For this review, take the finished solid that the model builds, in its own axes (mm). Face numbers are marked on the shaded views. A direction names the side the tool comes from. Round coordinates to 2 decimals unless told otherwise and drop trailing zeros. Order: outer loops, then holes, each group sorted by start corner. A loop starts at its lowest first (then second) coordinate and runs counter-clockwise, first axis right, second up. Notation, with made-up numbers: (-37.75, 54) -> (6.25, 54) arc R8 ccw to (6.25, 67) -> close; hole circle Ø7 at (22, 8). An arc over 180 degrees is marked (long way). Answer in a Markdown table with one row per item.
```python
from build123d import *

# Parameters (mm, degrees)
SKETCH_1_W               = 38.5
SKETCH_1_H               = 38.5
EXTRUDE_1_DEPTH          = 6.5
SKETCH_2_W               = 2.5
SKETCH_2_H               = 4
SKETCH_2_W_2             = 6
SKETCH_2_H_2             = 6
EXTRUDE_2_DEPTH          = 2
M3X0_5_1_D               = 2.5
M3X0_5_1_DEPTH           = 7.748924226
M3X0_5_1_TIP             = 0.751075774
CUT_EXTRUDE_1_DEPTH      = 3.5
PATTERN_CIRCULAR_1_COUNT = 4


with BuildPart() as part:
    # ｽｹｯﾁ1 → ﾎﾞｽ - 押し出し1 (new body)
    with BuildSketch(Plane.XY):
        Rectangle(SKETCH_1_W, SKETCH_1_H)
    extrude(amount=EXTRUDE_1_DEPTH)

    # ｽｹｯﾁ2 → ﾎﾞｽ - 押し出し2 (add)
    with BuildSketch(Plane.XY):
        with Locations((-20.5, 12.25)):
            Rectangle(SKETCH_2_W, SKETCH_2_H)
        with Locations((-20.5, 7.05)):
            Rectangle(SKETCH_2_W, SKETCH_2_H)
        with Locations((-20.5, 1.85)):
            Rectangle(SKETCH_2_W, SKETCH_2_H)
        with Locations((-20.5, -3.35)):
            Rectangle(SKETCH_2_W, SKETCH_2_H)
        with Locations((-20.5, -8.55)):
            Rectangle(SKETCH_2_W, SKETCH_2_H)
        with Locations((-20.5, -13.75)):
            Rectangle(SKETCH_2_W, SKETCH_2_H)
        with Locations((-3, -22.25)):
            Rectangle(SKETCH_2_W_2, SKETCH_2_H_2)
        with Locations((3, -22.25)):
            Rectangle(SKETCH_2_W_2, SKETCH_2_H_2)
        with Locations((20.5, -13.75)):
            Rectangle(SKETCH_2_W, SKETCH_2_H)
        with Locations((20.5, -8.55)):
            Rectangle(SKETCH_2_W, SKETCH_2_H)
        with Locations((20.5, 1.85)):
            Rectangle(SKETCH_2_W, SKETCH_2_H)
        with Locations((20.5, 7.05)):
            Rectangle(SKETCH_2_W, SKETCH_2_H)
        with Locations((20.5, 12.25)):
            Rectangle(SKETCH_2_W, SKETCH_2_H)
        with Locations((20.5, -3.35)):
            Rectangle(SKETCH_2_W, SKETCH_2_H)
    extrude(amount=EXTRUDE_2_DEPTH)

    # M3x0.5 ねじ穴1
    with Locations(Plane.XY.offset(6.5)):
        with Locations((-15, 15), (15, 15), (15, -15), (-15, -15)):
            Hole(M3X0_5_1_D / 2, depth=M3X0_5_1_DEPTH)
            with Locations((0, 0, -(M3X0_5_1_DEPTH + M3X0_5_1_TIP / 2))):  # 118° drill point
                Cone(0, M3X0_5_1_D / 2, M3X0_5_1_TIP, mode=Mode.SUBTRACT)

    # ｽｹｯﾁ5 → ｶｯﾄ - 押し出し1 (cut)
    with BuildSketch(Plane.XY.offset(6.5)):
        with BuildLine():
            Line((-11.5, 15), (-11.5, 19.25))
            Line((-11.5, 19.25), (-19.25, 19.25))
            Line((-19.25, 19.25), (-19.25, 11.5))
            Line((-19.25, 11.5), (-15, 11.5))
            ThreePointArc((-15, 11.5), (-12.525126266, 12.525126266), (-11.5, 15))
        make_face()
    cut_extrude_1 = extrude(amount=-CUT_EXTRUDE_1_DEPTH, mode=Mode.SUBTRACT)

    # 円形ﾊﾟﾀｰﾝ1: ｶｯﾄ - 押し出し1 ×4 about axis
    pattern_circular_1_axis = Axis((0, 0, 0), (0, 0, 1))
    for i in range(1, PATTERN_CIRCULAR_1_COUNT):
        add(cut_extrude_1.rotate(pattern_circular_1_axis, i * 360 / PATTERN_CIRCULAR_1_COUNT), mode=Mode.SUBTRACT)


solid = part.part
```
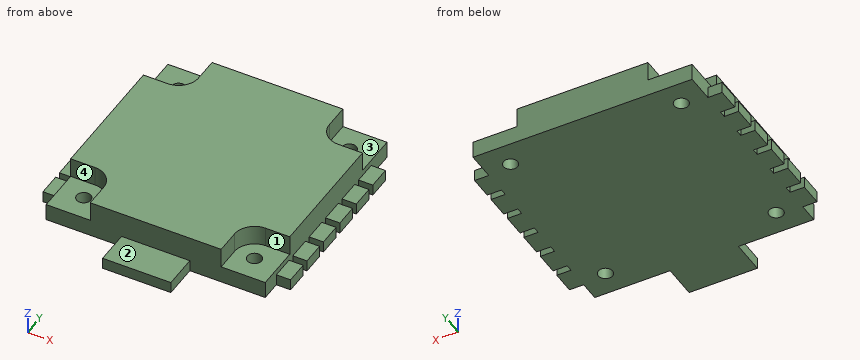
Q1. Tool access review of the marked faces 1, 2, 3 and 4: name each direction out of +Z, -Z, +X, -X, +Y, -Y from which nothing blocks a thin tool from reaching the whole face with its end or side.
Answer key:
| item | result |
|---|---|
| face 1 | +Z, +X, -Y |
| face 2 | +Z, +X, -X, -Y |
| face 3 | +Z, +X, +Y |
| face 4 | +Z, -X, -Y |
Q2. Clearance check with flat-ended pins moving along their axes: pin 1 Ø3 at (y, z) = (18, 5.5) entering from -X; pin 2 Ø3 at (x, y) = (20.5, 12.5) entering from +Z; pin 3 Ø1.2 at (x, y) = (-20, -3) entering from +Z. State where each tip first meets the part, or that it passes through.
Answer key:
| item | result |
|---|---|
| pin 1 | stops at x = -11.5 |
| pin 2 | stops at z = 3 |
| pin 3 | stops at z = 2 |
Q3. Take a section at B-B, the plane x = 1. Write out the cut boundary in (y, z).
Answer key:
| item | result |
|---|---|
| outline | (-25.25, 0) -> (19.25, 0) -> (19.25, 6.5) -> (-19.25, 6.5) -> (-19.25, 2) -> (-25.25, 2) -> close |
Q4. Take a section at C-C, the plane z = 0.75. Give the number of separate pieces and of enclosed holes in the cut face, then the cut area to 3 significant figures.
Answer key:
| item | result |
|---|---|
| separate pieces | 1 |
| enclosed holes | 4 |
| area | 1,650 mm^2 |
Q5. Take a section at A-A, the plane y = -18. Write out the cut boundary in (x, z).
Answer key:
| item | result |
|---|---|
| outline | (-19.25, 0) -> (19.25, 0) -> (19.25, 3) -> (11.5, 3) -> (11.5, 6.5) -> (-11.5, 6.5) -> (-11.5, 3) -> (-19.25, 3) -> close |
Q6. Take a section at D-D, the plane y = 3. Write out the cut boundary in (x, z).
Answer key:
| item | result |
|---|---|
| outline | (-21.75, 0) -> (21.75, 0) -> (21.75, 2) -> (19.25, 2) -> (19.25, 6.5) -> (-19.25, 6.5) -> (-19.25, 2) -> (-21.75, 2) -> close |
Q7. To check wall thickness, follow probe 1 along Y at (x, z) = (-15, 2); probe 2 along Y at (x, z) = (6, 5.25); probe 3 along Z at (x, y) = (-2, -20). State the ranges of each line that lie inside material, in increasing order.
Answer key:
| item | result |
|---|---|
| probe 1 | y = -19.25 to -16.25, -13.75 to 13.75, 16.25 to 19.25 |
| probe 2 | y = -19.25 to 19.25 |
| probe 3 | z = 0 to 2 |
